The figure shows three views and two pictorial views of one solid part (mm, origin at its lowest corner). Answer the questions. Round coordinates to 2 decimals unless told otherwise and drop trailing zeros. Order: outer loops, then holes, each group sorted by start corner. A loop starts at its lowest first (then second) coordinate and runs counter-clockwise, first axis right, second up. Notation, with made-up numbers: M -22,57 L 23,57 A30 ccw 23,80 Z; hole C -17,-34 d11. An arc over 180 degrees is marked long. Return JSON: item names as keys, results as strings.
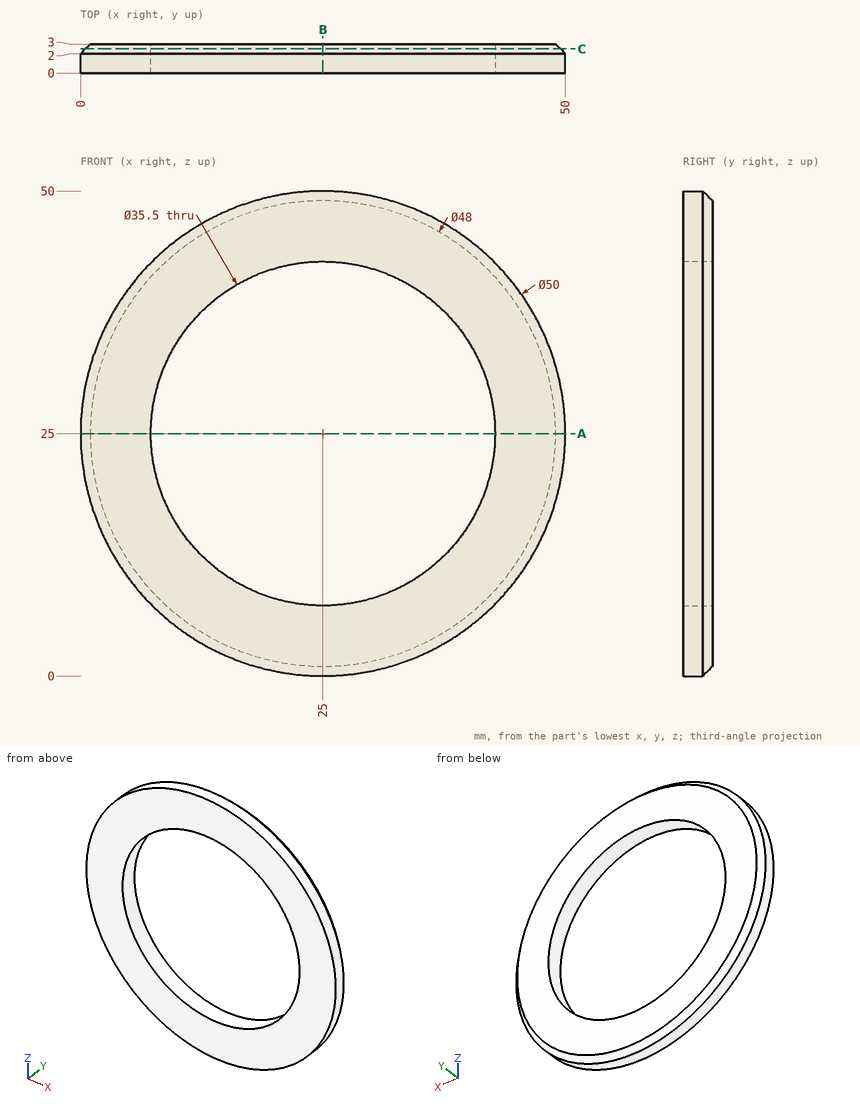
Item 1: Find section B-B (x = 25). Determine the outline of the cut face in (y, z), plus the area to 3 significant figures.
Output:
{"outline": "M 0,0 L 2,0 L 3,1 L 3,7.25 L 0,7.25 Z; M 0,42.75 L 3,42.75 L 3,49 L 2,50 L 0,50 Z", "area": "42.5 mm^2"}
Item 2: Consider line 1 along X through (y, z) = (0.65, 25); line 2 along X through (y, z) = (0.25, 27). Determine where each line is inside the solid, lowest interval first. Write a range as [from, to].
Output:
{"line 1": "x = [0, 7.25], [42.75, 50]", "line 2": "x = [0.08, 7.36], [42.64, 49.92]"}
Item 3: This flat-tipped pin is pushed along its axis until it touches: pin 1 (1.5 mm diameter, centred on y = 1, z = 43, fed in from -X). Where does it stop, or does it pass through?
Output:
{"pin 1": "stops at x = 6.9"}
Item 4: Find section C-C (y = 2.5). Determine the outline of the cut face in (x, z), plus the area to 3 significant figures.
Output:
{"outline": "C 25,25 d49; hole C 25,25 d35.5", "area": "896 mm^2"}
Item 5: Find section A-A (z = 25). Determine the outline of the cut face in (x, y).
Output:
{"outline": "M 0,0 L 7.25,0 L 7.25,3 L 1,3 L 0,2 Z; M 42.75,0 L 50,0 L 50,2 L 49,3 L 42.75,3 Z"}
